Autodesk Inventor part; units mm, degrees
ref_plane "YZ Plane" through (0, 0, 0) normal (1, 0, 0) x (0, 1, 0)
ref_plane "XZ Plane" through (0, 0, 0) normal (0, 1, 0) x (-1, 0, 0)
ref_plane "XY Plane" through (0, 0, 0) normal (0, 0, 1) x (1, 0, 0)
sketch "スケッチ1" plane through (0, 0, 0) normal (0, 1, 0) x (-1, 0, 0)
  circle A0 centre (0, 0) radius 1
  circle A1 centre (0, 0) radius 3.5
  circle A2 centre (-8.2843, 0) radius 3.5
  line L0 (0, -3.5) -> (-8.2843, -3.5)
  line L1 (-8.2843, -3.5) -> (-8.2843, 3.5) construction
  line L2 (-8.2843, 3.5) -> (0, 3.5)
  line L3 (0, 3.5) -> (0, -3.5) construction
  circle A3 centre (-8.2843, 0) radius 1
  line L4 (-3.5, -3.5) -> (-4.7843, -3.5)
  line L5 (-4.7843, -3.5) -> (-4.7843, 3.5)
  line L6 (-4.7843, 3.5) -> (-3.5, 3.5)
  line L7 (-3.5, 3.5) -> (-3.5, -3.5)
  circle A4 centre (-4.1421, 10) radius 10
  line L8 (0, 0) -> (-8.2843, 0)
  line L9 (-4.1421, 10) -> (0, 0)
  line L10 (-4.1421, 10) -> (-8.2843, 0)
  point P0 (-8.2843, -3.5)
  point P1 (-4.7843, -3.5)
  point P2 (-4.1421, 0)
  dimension "d1" = 7
  dimension "d0" = 2
  dimension "d13" = 20
  dimension "d14" = 45
extrude "押し出し3" add sketch "スケッチ1" along normal blind 5 contours A0 A4 A1 L8 | A0 L9 A1 A4 | L8 A4 A0 | A0 A4 A1 L9 | L7 L2 L9 A1 | A4 L5 L2 L7 | A1 L0 L7 | L7 L0 L5 L8 A4 | L9 L2 A1 | L8 A2 A4 | A4 A3 L8 A2 | A2 L10 A3 A4 | L5 A2 L10 L2 | L0 A2 L5 | A4 A3 L10 A2 | A2 L8 A3 A4 | L2 L10 A2
extrude "押し出し4" cut sketch "スケッチ1" along normal blind 2.1 contours A0 A4 A1 L8 | A0 L9 A1 A4 | L8 A4 A0 | A0 A4 A1 L9 | L7 L2 L9 A1 | A1 L0 L7 | L9 L2 A1 | A4 A3 L8 A2 | A2 L10 A3 A4 | L5 A2 L10 L2 | L0 A2 L5 | A4 A3 L10 A2 | A2 L8 A3 A4 | L2 L10 A2
mirror "ミラー2" about plane through (4.1421, 0, 0) normal (0, -1, 0)
sketch "スケッチ3" plane through (0, 5, 0) normal (0, 1, 0) x (1, 0, 0)
  circle A0 centre (14.2843, 0) radius 1.35
  line L0 (4.7843, -3.5) -> (8.2843, -3.5)
  line L1 (8.2843, -3.5) -> (17.7843, -3.5)
  line L2 (17.7843, -3.5) -> (17.7843, 3.5)
  line L3 (17.7843, 3.5) -> (8.2843, 3.5)
  line L4 (8.2843, 3.5) -> (8.2843, -3.5)
  line L5 (8.2843, 3.5) -> (0, 3.5)
  circle A1 centre (14.2843, 0) radius 3.5
  line L6 (4.7843, -3.5) -> (8.2843, -3.5)
  line L7 (4.7843, 3.5) -> (4.7843, -3.5)
  line L8 (8.2843, 3.5) -> (4.7843, 3.5)
  arc A2 (8.2843, -3.5) -> (8.2843, 3.5) centre (8.2843, 0) ccw
  circle A3 centre (8.2843, 0) radius 1
  point P0 (0, 0)
  point P1 (8.2843, 0)
  point P2 (14.2843, -3.5)
  point P3 (14.2843, 3.5)
  dimension "d15" = 2.7
  dimension "d16" = 6
extrude "押し出し5" add sketch "スケッチ3" against normal up to surface (10 mm away) contours L7 L5 L4 A3 L0 | L4 A3 A2 A1 | A1 A2 picked at (11.1245, 0.126)
sketch "スケッチ4" plane through (0, 5, 0) normal (0, 1, 0) x (1, 0, 0)
  circle A0 centre (8.2843, 0) radius 1
  circle A1 centre (8.2843, 0) radius 1.35
  point P0 (0, 0)
  dimension "d20" = 2.7
extrude "押し出し6" cut sketch "スケッチ4" against normal through all contours A0 | A1
sketch "スケッチ5" plane through (0, 5, 0) normal (0, 1, 0) x (1, 0, 0)
  circle A0 centre (8.2843, 0) radius 1.35
  circle A1 centre (0, 0) radius 1
  arc A2 (0, 3.5) -> (0, -3.5) centre (0, 0) ccw
  line L0 (0, -3.5) -> (8.2843, -3.5)
  circle A3 centre (8.2843, 0) radius 3.5
  line L1 (8.2843, 3.5) -> (0, 3.5)
  arc A4 (8.2843, -3.5) -> (8.2843, 3.5) centre (8.2843, 0) ccw
  point P0 (8.2843, -3.5)
  point P1 (8.2843, -3.5)
extrude "押し出し7" add sketch "スケッチ5" along normal blind 1 contours A3
properties part number "chain_fork_connector"
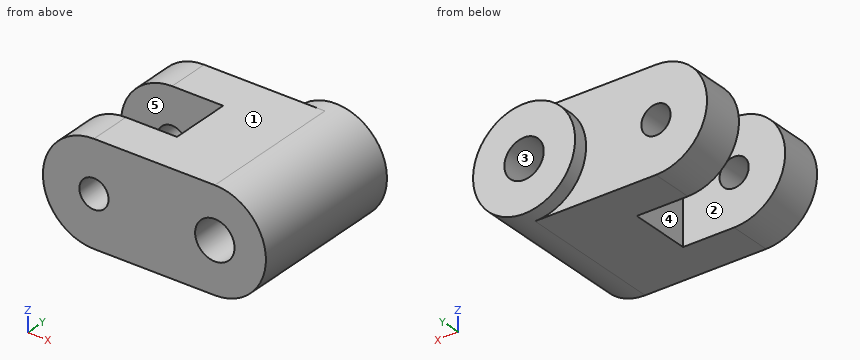
For this review, take the finished solid that the model builds, in its own axes (mm). Face numbers are marked on the shaded views. A direction names the side the tool comes from. Coordinates: 2 decimals unless noted, no trailing zeros. Write each loop counter-clockwise with the first axis right and the second up, starting at its lowest first coordinate (ties: lowest second). Pieces come first, ordered by that corner, then holes.
(1) Add section D-D on y = -0.75. Give the boundary of the cut face in (x, z), then the cut area to 3 significant figures.
(2) Add section B-B on y = -3.75. Give the boundary of the cut face in (x, z).
(3) The part is to be moulded in two halves that separate along X. For the marked faces 3, 4 and 5, say which applies: +X half, -X half, draft (parallel to the pull), parting line (faces both ways), or undercut.
(4) Add section C-C on z = 0.75. Give the boundary of the cut face in (x, y).
(5) Tool access review of the marked faces 1 and 2: name each direction out of +Z, -Z, +X, -X, +Y, -Y from which nothing blocks a thin tool from reaching the whole face with its end or side.
(6) Add section A-A on x = 1.5. Give the boundary of the cut face in (y, z), then the cut area to 3 significant figures.
(7) For pin 1 Ø3 at (y, z) = (-3, 2.5) entering from +X; pin 2 Ø3.5 at (x, z) = (0.5, -0.5) entering from +Y; pin 3 Ø1.2 at (x, z) = (0, 0) entering from -Y, all flat-tipped, find the tip position at first contact; note any pin that passes through.
(8) Wall thickness on probe 1 along Y at (x, z) = (0, 3); probe 2 along Z at (x, y) = (8.5, 3.5); probe 3 along Z at (x, y) = (9, 0.25): over which ranges is each line inside the solid? List them lowest first.
Answer sheet:
1. outline: (3.5, -3.5) - (8.28, -3.5) arc R3.5 ccw to (8.28, 3.5) - (3.5, 3.5) - close; hole circle Ø2.7 at (8.28, 0)
1. area: 47.0 mm2
2. outline: (0, -3.5) - (8.28, -3.5) arc R3.5 ccw to (8.28, 3.5) - (0, 3.5) arc R3.5 ccw to start; hole circle Ø2 at (0, 0); hole circle Ø2.7 at (8.28, 0)
3. face 3: undercut
3. face 4: -X half
3. face 5: draft
4. outline: (-3.42, -5) - (-0.66, -5) - (-0.66, -2.1) - (-3.42, -2.1) - close; (-3.42, 2.1) - (-0.66, 2.1) - (-0.66, 5) - (-3.42, 5) - close; (0.66, -5) - (7.16, -5) - (7.16, 6) - (4.87, 6) - (4.87, 5) - (0.66, 5) - (0.66, 2.1) - (3.5, 2.1) - (3.5, -2.1) - (0.66, -2.1) - close; (9.41, -5) - (11.7, -5) - (11.7, 6) - (9.41, 6) - close
5. face 1: +Z, +X, -X, +Y, -Y
5. face 2: +Z, -Z, -X
6. outline: (-5, -3.5) - (-2.1, -3.5) - (-2.1, 3.5) - (-5, 3.5) - close; (2.1, -3.5) - (5, -3.5) - (5, 3.5) - (2.1, 3.5) - close
6. area: 40.6 mm2
7. pin 1: stops at x = 11.64
7. pin 2: stops at y = 5
7. pin 3: passes through
8. probe 1: y = -5 to -2.1, 2.1 to 5
8. probe 2: z = -3.49 to -1.33, 1.33 to 3.49
8. probe 3: z = -3.43 to -1.14, 1.14 to 3.43
